Geometry check sheet. Reference: the model listing, model coordinates, mm. Round coordinates to 2 decimals unless told otherwise and drop trailing zeros. Order: outer loops, then holes, each group sorted by start corner. A loop starts at its lowest first (then second) coordinate and runs counter-clockwise, first axis right, second up.
(1) Sectioned sample at A-A (z = 22.5). Record the boundary of the cut face in (x, y) (3 decimals).
(2) Sectioned sample at B-B (y = 0). Record the boundary of the cut face in (x, z) (3 decimals), plus the area to 3 significant figures.
(3) Go/stop test with flat-tipped pins: pin 1 (3 mm diameter, centred on y = -3, z = 5.5, fed in from -X); pin 2 (4 mm diameter, centred on x = -4.5, z = 13.5, fed in from -Y) (3 decimals); pin 3 (6 mm diameter, centred on x = 0, z = 26, fed in from +Y) (3 decimals); pin 4 (12 mm diameter, centred on x = 1, z = 11.5, fed in from +Y) (3 decimals). Record where each tip stops, or that it passes through.
(4) Release check for a two-part mould opening along X. For faces 1 (the face through (17.125, 0, 26)), 2 (the face through (8.7, -13.5, 21)), 3 (the face through (0, -10.125, 15)), 4 (the face through (-16.946, 14.571, 26.063)) record: +X half, -X half, draft (parallel to the pull), parting line (faces both ways), or undercut.
(5) Sectioned sample at C-C (x = 0). Give the number of separate pieces and of enclosed holes in the cut face, plus the area to 3 significant figures.
(6) Material ranges on line 1 along Y through (x, z) = (4, 27.5) (3 decimals); line 2 along Y through (x, z) = (4, 4) (3 decimals), recorded low to high.
from build123d import *

# Parameters (mm, degrees)
SKIZZE1_R                       = 15.725
SKIZZE1_W                       = 20.25
SKIZZE1_H                       = 20.25
AUFSATZ_LINEAR_AUSTRAGEN1_DEPTH = 21
SKIZZE2_W                       = 20.25
SKIZZE2_H                       = 20.25
AUFSATZ_LINEAR_AUSTRAGEN2_DEPTH = 10
SKIZZE3_R                       = 2.3
SCHNITT_LINEAR_AUSTRAGEN1_DEPTH = 50.267921866
VERRUNDUNG1_R                   = 0.2
VERRUNDUNG2_R                   = 2.5
FASE1_SIZE                      = 0.5
FASE4_SIZE                      = 0.5


with BuildPart() as part:
    # Skizze1 → Aufsatz-Linear austragen1 (new body)
    with BuildSketch(Plane.XY):
        with Locations(Location((0, 0, 0), (0, 0, 180))):
            Circle(SKIZZE1_R)
        Rectangle(SKIZZE1_W, SKIZZE1_H, mode=Mode.SUBTRACT)
    extrude(amount=AUFSATZ_LINEAR_AUSTRAGEN1_DEPTH)

    # Skizze2 → Aufsatz-Linear austragen2 (add)
    with BuildSketch(Plane.XY.offset(21)):
        with BuildLine():
            Line((-14.593984206, 17.125), (14.593984206, 17.125))
            ThreePointArc((14.593984206, 17.125), (15.909902577, 15.909902577), (17.125, 14.593984206))
            Line((17.125, 14.593984206), (17.125, -14.593984206))
            ThreePointArc((17.125, -14.593984206), (15.909902577, -15.909902577), (14.593984206, -17.125))
            Line((14.593984206, -17.125), (-14.593984206, -17.125))
            ThreePointArc((-14.593984206, -17.125), (-15.909902577, -15.909902577), (-17.125, -14.593984206))
            Line((-17.125, -14.593984206), (-17.125, 14.593984206))
            ThreePointArc((-17.125, 14.593984206), (-15.909902577, 15.909902577), (-14.593984206, 17.125))
        make_face()
        Rectangle(SKIZZE2_W, SKIZZE2_H, mode=Mode.SUBTRACT)
    extrude(amount=AUFSATZ_LINEAR_AUSTRAGEN2_DEPTH)

    # Skizze3 → Schnitt-Linear austragen1 (cut, through all)
    with BuildSketch(Plane(origin=(0, 17.125, 0), x_dir=(1, 0, 0), z_dir=(0, 1, 0))):
        with Locations(Location((0, -26, 0), (0, 0, 270))):
            Circle(SKIZZE3_R)
    extrude(amount=-SCHNITT_LINEAR_AUSTRAGEN1_DEPTH, mode=Mode.SUBTRACT)

    # Verrundung1
    verrundung1_edges = [part.edges().sort_by_distance(p)[0] for p in [
        (10.125, -10.125, 15.5),
        (10.125, 10.125, 15.5),
        (-10.125, 10.125, 15.5),
        (-10.125, -10.125, 15.5),
    ]]
    fillet(verrundung1_edges, radius=VERRUNDUNG1_R)

    # Verrundung2
    verrundung2_edges = [part.edges().sort_by_distance(p)[0] for p in [
        (-14.593984206, 17.125, 26),
        (-17.125, 14.593984206, 26),
        (-17.125, -14.593984206, 26),
        (-14.593984206, -17.125, 26),
        (14.593984206, -17.125, 26),
        (17.125, -14.593984206, 26),
        (17.125, 14.593984206, 26),
        (14.593984206, 17.125, 26),
    ]]
    fillet(verrundung2_edges, radius=VERRUNDUNG2_R)

    # Fase1
    fase1_edges = [part.edges().sort_by_distance(p)[0] for p in [
        (0, 17.125, 31),
        (-14.558620883, 16.950974258, 31),
        (-16.950974258, 14.558620883, 31),
        (14.558620883, 16.950974258, 31),
        (16.950974258, 14.558620883, 31),
        (16.950974258, -14.558620883, 31),
        (14.558620883, -16.950974258, 31),
        (-14.558620883, -16.950974258, 31),
        (-16.950974258, -14.558620883, 31),
        (15.725, 0, 0),
        (0, -10.125, 23.7),
        (0, 10.125, 23.7),
        (0, -17.125, 23.7),
        (0, 17.125, 23.7),
        (0, -10.125, 0),
        (0, -10.125, 31),
        (10.125, 0, 0),
        (10.125, 0, 31),
        (-10.125, 0, 0),
        (-10.125, 0, 31),
        (0, 10.125, 0),
        (0, 10.125, 31),
        (10.066421356, -10.066421356, 0),
        (10.066421356, -10.066421356, 31),
        (-10.066421356, -10.066421356, 0),
        (-10.066421356, -10.066421356, 31),
        (-10.066421356, 10.066421356, 0),
        (-10.066421356, 10.066421356, 31),
        (10.066421356, 10.066421356, 0),
        (10.066421356, 10.066421356, 31),
        (-15.909902577, -15.909902577, 31),
        (-17.125, 0, 31),
        (-15.909902577, 15.909902577, 31),
        (0, -17.125, 31),
        (15.909902577, -15.909902577, 31),
        (17.125, 0, 31),
        (15.909902577, 15.909902577, 31),
    ]]
    chamfer(fase1_edges, length=FASE1_SIZE)

    # Fase4
    fase4_edges = [part.edges().sort_by_distance(p)[0] for p in [
        (-15.909902577, -15.909902577, 21),
        (-15.909902577, 15.909902577, 21),
        (0, 17.125, 21),
        (15.909902577, 15.909902577, 21),
        (17.125, 0, 21),
        (15.909902577, -15.909902577, 21),
        (0, -17.125, 21),
        (-17.125, 0, 21),
        (-14.558620883, 16.950974258, 21),
        (-16.950974258, 14.558620883, 21),
        (14.558620883, 16.950974258, 21),
        (16.950974258, 14.558620883, 21),
        (16.950974258, -14.558620883, 21),
        (14.558620883, -16.950974258, 21),
        (-14.558620883, -16.950974258, 21),
        (-16.950974258, -14.558620883, 21),
    ]]
    chamfer(fase4_edges, length=FASE4_SIZE)


solid = part.part
Answer below:
1. outline: (-17.125, -13.642) arc R2.5 ccw to (-16.453, -15.347) arc R22.5 ccw to (-15.347, -16.453) arc R2.5 ccw to (-13.642, -17.125) - (13.642, -17.125) arc R2.5 ccw to (15.347, -16.453) arc R22.5 ccw to (16.453, -15.347) arc R2.5 ccw to (17.125, -13.642) - (17.125, 13.642) arc R2.5 ccw to (16.453, 15.347) arc R22.5 ccw to (15.347, 16.453) arc R2.5 ccw to (13.642, 17.125) - (-13.642, 17.125) arc R2.5 ccw to (-15.347, 16.453) arc R22.5 ccw to (-16.453, 15.347) arc R2.5 ccw to (-17.125, 13.642) - close; hole (-10.125, -9.925) arc R0.2 ccw to (-9.925, -10.125) - (9.925, -10.125) arc R0.2 ccw to (10.125, -9.925) - (10.125, 9.925) arc R0.2 ccw to (9.925, 10.125) - (-9.925, 10.125) arc R0.2 ccw to (-10.125, 9.925) - close
2. outline: (-17.125, 21.5) - (-16.625, 21) - (-15.725, 21) - (-15.725, 0.5) - (-15.225, 0) - (-10.625, 0) - (-10.125, 0.5) - (-10.125, 30.5) - (-10.625, 31) - (-16.625, 31) - (-17.125, 30.5) - close; (10.125, 0.5) - (10.625, 0) - (15.225, 0) - (15.725, 0.5) - (15.725, 21) - (16.625, 21) - (17.125, 21.5) - (17.125, 30.5) - (16.625, 31) - (10.625, 31) - (10.125, 30.5) - close
2. area: 374 mm2
3. pin 1: stops at x = -15.65
3. pin 2: stops at y = -15.525
3. pin 3: stops at y = 17.125
3. pin 4: stops at y = 15.725
4. face 1: +X half
4. face 2: draft
4. face 3: undercut
4. face 4: -X half
5. separate pieces: 4
5. enclosed holes: 0
5. area: 309 mm2
6. line 1: y = -17.125 to -10.125, 10.125 to 17.125
6. line 2: y = -15.208 to -10.125, 10.125 to 15.208
